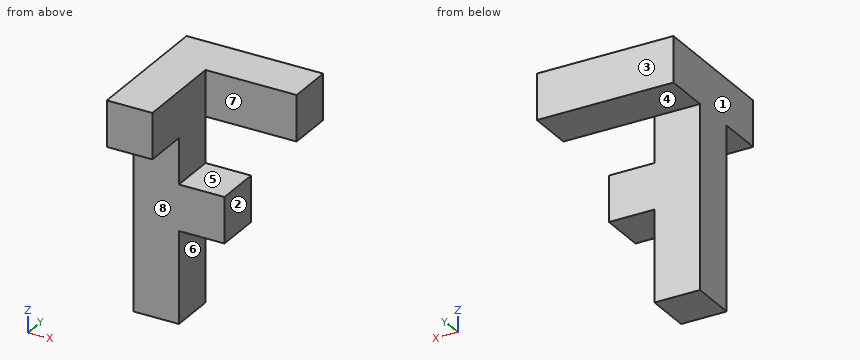
```python
from build123d import *

# Parameters (mm, degrees)
F0_W          = 12.7
F0_H          = 12.7
F1_DEPTH      = 12.7
F2_W          = 12.7
F2_H          = 12.7
F3_DEPTH      = 12.7
F3_DEPTH_BACK = 25.4
F4_W          = 12.7
F4_H          = 12.7
F5_DEPTH      = 25.4


with BuildPart() as f1:
    # F0 (on Front) → F1 (new body)
    with BuildSketch(Plane.XZ):
        Polygon((0, 63.5), (0, 0), (12.7, 0), (12.7, 25.4), (12.7, 38.1), (12.7, 63.5), align=None)
        with Locations((19.05, 31.75)):
            Rectangle(F0_W, F0_H)
    extrude(amount=F1_DEPTH)

    # F2 (on face) → F3 (join, two sides)
    with BuildSketch(Plane.XZ.offset(12.7)) as f3_sk:
        with Locations((6.35, 57.15)):
            Rectangle(F2_W, F2_H)
    extrude(amount=F3_DEPTH)
    extrude(f3_sk.sketch, amount=-F3_DEPTH_BACK)

    # F4 (on face) → F5 (join)
    with BuildSketch(Plane.YZ.offset(12.7)):
        with Locations((6.35, 57.15)):
            Rectangle(F4_W, F4_H)
    extrude(amount=F5_DEPTH)


solid = f1.part
```
Source: CAD feature listing. Evaluate the final solid. Frame: model axes, mm. Face numbers are marked on the shaded views. A direction names the side the tool comes from. Coordinates: 2 decimals unless noted, no trailing zeros. Loops run counter-clockwise (first coordinate to the right, second up) from the corner with the lowest first, then second, coordinate; pieces in that order, holes last. Notation, with made-up numbers: (33.25, 23.25) -> (70.25, 23.25) arc R21 ccw to (70.25, 31.25) -> close; hole circle Ø6 at (59.5, -1.5). An arc over 180 degrees is marked (long way). One line per item, written item: value. Start each with the question number.
Q1. Section query D-D, the plane z = 58. Return the cut outline in (x, y).
Q2. Line query: line 1 along Y through (x, z) = (23, 27.5); line 2 along X through (y, z) = (-11.5, 52); line 3 along Z through (x, y) = (5.5, 10.5). Output: solid intervals per line, ascending.
Q3. Mould query, pull axis X, two halves, no side actions, for the marked faces 1, 2 and 3. Classes: pulls with the +X half, pulls with the -X half, needs draft (parallel to the pull), parting line crosses it, or undercut.
Q4. Contact query for flat-ended pins moving along their axis: P1, Ø14, axis at y = -7.5, z = 6.5, coming from the +X side; P2, Ø6.5, axis at x = 4.5, y = -17.5, coming from the -Z side; P3, Ø6.5, axis at x = 18, y = -5, coming from the -Z side. Output: stop coordinate, or through.
Q5. Set-up query: the marked faces 4, 5, 6, 7 and 8. Return all of +Z, -Z, +X, -X, +Y, -Y with unobstructed straight access to the full face (end or side cutting, diameter ignored); none if empty.
Q6. Section query A-A, the plane x = 20.5. Return the cut outline in (y, z).
Q7. Section query C-C, the plane x = 7. Return the cut outline in (y, z).
Q8. Section query B-B, the plane y = -9.5. Return the cut outline in (x, z), and give its area (3 significant figures).
Results:
1. outline: (0, -25.4) -> (12.7, -25.4) -> (12.7, 0) -> (38.1, 0) -> (38.1, 12.7) -> (0, 12.7) -> close
2. line 1: -12.7 to 0
2. line 2: 0 to 12.7
2. line 3: 50.8 to 63.5
3. face 1: pulls with the -X half
3. face 2: pulls with the +X half
3. face 3: needs draft
4. P1: x = 12.7
4. P2: z = 50.8
4. P3: z = 25.4
5. face 4: -Z, +X, -X, +Y
5. face 5: +Z, +X, +Y, -Y
5. face 6: -Z, +X, +Y, -Y
5. face 7: +Z, +X, -Y
5. face 8: -Z, +X, -X, -Y
6. outline: (-12.7, 25.4) -> (0, 25.4) -> (0, 38.1) -> (-12.7, 38.1) -> close; (0, 50.8) -> (12.7, 50.8) -> (12.7, 63.5) -> (0, 63.5) -> close
7. outline: (-25.4, 50.8) -> (-12.7, 50.8) -> (-12.7, 0) -> (0, 0) -> (0, 50.8) -> (12.7, 50.8) -> (12.7, 63.5) -> (-25.4, 63.5) -> close
8. outline: (0, 0) -> (12.7, 0) -> (12.7, 25.4) -> (25.4, 25.4) -> (25.4, 38.1) -> (12.7, 38.1) -> (12.7, 63.5) -> (0, 63.5) -> close
8. area: 968 mm^2
